Read the model definition and answer for the solid it produces. Units are mm, in the model's axes. Face numbers are marked on the shaded views. A direction names the side the tool comes from. Coordinates: 2 decimals unless noted, no trailing zeros. Order: outer loops, then holes, each group sorted by start corner. A loop starts at its lowest first (then second) coordinate and runs counter-clockwise, first axis right, second up. Notation, with made-up numbers: (52.5, -2.75) -> (105.5, -2.75) arc R18 cw to (105.5, 21.25) -> close; hole circle Ø6 at (-8.5, -17). An arc over 180 degrees is marked (long way). Answer as a JSON object with one key per item and string values. Group by question number.
1) Section D-D on y = 10.5 is taken. Determine the outline of the cut face in (x, z).
2) Consider L1, parallel to Z at x = 5, y = 23; L2, parallel to Y at x = 10.5, z = -26; L3, parallel to Y at x = -13, z = -24.5. Determine where each line is inside the solid, lowest interval first.
3) A tool of negligible diameter and unlimited length cuts with its end or side. For the marked faces 4 and 5, from which of +Z, -Z, +X, -X, +Y, -Y can it reach the whole face along a straight path? Write none if from no direction.
4) Determine the mould class of the marked faces 1, 2 and 3 for opening direction Z: released by +Z, released by -Z, zero draft, split by the parting line, or undercut.
5) Section C-C on z = 26 is taken. Determine the outline of the cut face in (x, y), and give its area (3 significant figures).
6) Section A-A on z = -10 is taken. Determine the outline of the cut face in (x, y).
7) Section B-B on x = -16.5 is taken. Determine the outline of the cut face in (y, z), and give its area (3 significant figures).
8) Given pin 1 (6 mm diameter, centred on y = 34.5, z = -14, fed in from -X); pin 2 (1.7 mm diameter, centred on y = 59, z = 9, fed in from -X); pin 3 (0.8 mm diameter, centred on y = 20, z = 29, fed in from -X), each flat-ended and moving along its own axis, determine where each tip first touches the part or whether it passes through.
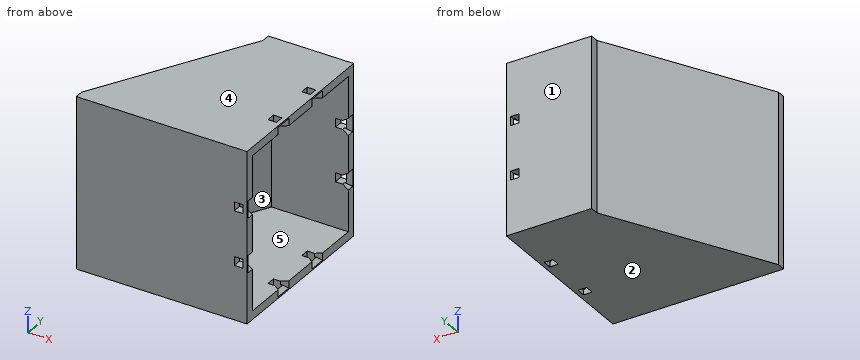
from build123d import *

# Parameters (mm, degrees)
SKETCH_1_W                    = 60
SKETCH_1_H                    = 60
EXTRUDE_1_DEPTH               = 3
SKETCH_2_W                    = 30
SKETCH_2_H                    = 60
EXTRUDE_2_DEPTH               = 3
EXTRUDE_3_DEPTH               = 3
EXTRUDE_4_DEPTH               = 3
SKETCH_8_W                    = 3
SKETCH_8_H                    = 3.1
CUT_EXTRUDE_2_DEPTH           = 91.000000167
SKETCH_9_W                    = 3
SKETCH_9_H                    = 3.1
CUT_EXTRUDE_3_DEPTH           = 74.484692447
SKETCH_7_W                    = 6
SKETCH_7_H                    = 5
CUT_EXTRUDE_1_DEPTH           = 2
CUT_EXTRUDE_1_DRAFT           = -36
SKETCH_7_W_2                  = 5
SKETCH_7_H_2                  = 6
CUT_EXTRUDE_1_PROFILE_2_DEPTH = 2
CUT_EXTRUDE_1_PROFILE_2_DRAFT = -36
CUT_EXTRUDE_1_PROFILE_3_DEPTH = 2
CUT_EXTRUDE_1_PROFILE_3_DRAFT = -36
CUT_EXTRUDE_1_PROFILE_4_DEPTH = 2
CUT_EXTRUDE_1_PROFILE_4_DRAFT = -36
CUT_EXTRUDE_1_PROFILE_5_DEPTH = 2
CUT_EXTRUDE_1_PROFILE_5_DRAFT = -36
CUT_EXTRUDE_1_PROFILE_6_DEPTH = 2
CUT_EXTRUDE_1_PROFILE_6_DRAFT = -36
CUT_EXTRUDE_1_PROFILE_7_DEPTH = 2
CUT_EXTRUDE_1_PROFILE_7_DRAFT = -36
CUT_EXTRUDE_1_PROFILE_8_DEPTH = 2
CUT_EXTRUDE_1_PROFILE_8_DRAFT = -36


with BuildPart() as part:
    # Sketch 1 → Extrude 1 (new body)
    with BuildSketch(Plane(origin=(0, 0, 0), x_dir=(1, 0, 0), z_dir=(0, 1, 0))):
        Rectangle(SKETCH_1_W, SKETCH_1_H)
    extrude(amount=EXTRUDE_1_DEPTH)



with BuildPart() as body_2:
    # Sketch 2 → Extrude 2 (new body)
    with BuildSketch(Plane(origin=(0, 57, 0), x_dir=(1, 0, 0), z_dir=(0, 1, 0))):
        with Locations((15, 0)):
            Rectangle(SKETCH_2_W, SKETCH_2_H)
    extrude(amount=EXTRUDE_2_DEPTH)


with BuildPart() as part_1:
    add(part.part)

    add(body_2.part)  # Loft 1 merges body 2
    # Sketch 3 → Loft 1 section 0
    with BuildSketch(Plane.XZ.offset(-57)):
        with BuildLine():
            Line((0, 30), (3, 30))
            Line((3, 30), (3, -30))
            Line((3, -30), (0, -30))
            Line((0, -30), (0, 30))
        make_face()
    # Sketch 4 → Loft 1 section 1
    with BuildSketch(Plane(origin=(0, 3, 0), x_dir=(1, 0, 0), z_dir=(0, 1, 0))):
        with BuildLine():
            Line((-30, 30), (-27, 30))
            Line((-27, 30), (-27, -30))
            Line((-27, -30), (-30, -30))
            Line((-30, -30), (-30, 30))
        make_face()
    loft()

    # Sketch 5 → Extrude 3 (add)
    with BuildSketch(Plane.XY.offset(30)):
        Polygon((30, 57), (3, 57), (-27, 3), (30, 3), align=None)
    extrude(amount=-EXTRUDE_3_DEPTH)

    # Sketch 6 → Extrude 4 (add)
    with BuildSketch(Plane(origin=(0, 0, -30), x_dir=(-1, 0, 0), z_dir=(0, 0, -1))):
        Polygon((-30, 57), (-3, 57), (27, 3), (-30, 3), align=None)
    extrude(amount=-EXTRUDE_4_DEPTH)

    # Sketch 8 → Cut-Extrude 2 (cut, through all)
    with BuildSketch(Plane(origin=(0, 0, -30), x_dir=(-1, 0, 0), z_dir=(0, 0, -1))):
        with Locations((-27, 39.5)):
            Rectangle(SKETCH_8_W, SKETCH_8_H)
        with Locations((-27, 20.5)):
            Rectangle(SKETCH_8_W, SKETCH_8_H)
    extrude(amount=-CUT_EXTRUDE_2_DEPTH, mode=Mode.SUBTRACT)

    # Sketch 9 → Cut-Extrude 3 (cut, through all)
    with BuildSketch(Plane(origin=(0, 60, 0), x_dir=(1, 0, 0), z_dir=(0, 1, 0))):
        with Locations((27, 9.5)):
            Rectangle(SKETCH_9_W, SKETCH_9_H)
        with Locations((27, -9.5)):
            Rectangle(SKETCH_9_W, SKETCH_9_H)
    extrude(amount=-CUT_EXTRUDE_3_DEPTH, mode=Mode.SUBTRACT)


with BuildPart() as cut_extrude_1_tool:
    # Sketch 7 → Cut-Extrude 1 (with draft: the straight prism first)
    with BuildSketch(Plane(origin=(30, 0, 0), x_dir=(0, 0, -1), z_dir=(1, 0, 0))):
        with Locations((9.5, 3)):
            Rectangle(SKETCH_7_W, SKETCH_7_H)
    extrude(amount=-CUT_EXTRUDE_1_DEPTH)
    # Cut-Extrude 1: the draft: its side faces are tilted about the plane it starts from
    cut_extrude_1_sides = [cut_extrude_1_tool.faces().sort_by_distance(p)[0] for p in [
        (29, 3, -6.5),
        (29, 0.5, -9.5),
        (29, 3, -12.5),
        (29, 5.5, -9.5),
    ]]
    draft(cut_extrude_1_sides, Plane(origin=(30, 0, 0), x_dir=(0, 0, -1), z_dir=(1, 0, 0)), CUT_EXTRUDE_1_DRAFT)


with BuildPart() as part_2:
    add(part_1.part)

    # Cut-Extrude 1: cut by cut_extrude_1_tool
    add(cut_extrude_1_tool.part, mode=Mode.SUBTRACT)


with BuildPart() as cut_extrude_1_profile_2_tool:
    # Sketch 7 → Cut-Extrude 1 profile 2 (with draft: the straight prism first)
    with BuildSketch(Plane(origin=(30, 0, 0), x_dir=(0, 0, -1), z_dir=(1, 0, 0))):
        with Locations((27, 39.5)):
            Rectangle(SKETCH_7_W_2, SKETCH_7_H_2)
    extrude(amount=-CUT_EXTRUDE_1_PROFILE_2_DEPTH)
    # Cut-Extrude 1 profile 2: the draft: its side faces are tilted about the plane it starts from
    cut_extrude_1_profile_2_sides = [cut_extrude_1_profile_2_tool.faces().sort_by_distance(p)[0] for p in [
        (29, 36.5, -27),
        (29, 39.5, -29.5),
        (29, 42.5, -27),
        (29, 39.5, -24.5),
    ]]
    draft(cut_extrude_1_profile_2_sides, Plane(origin=(30, 0, 0), x_dir=(0, 0, -1), z_dir=(1, 0, 0)), CUT_EXTRUDE_1_PROFILE_2_DRAFT)


with BuildPart() as part_3:
    add(part_2.part)

    # Cut-Extrude 1 profile 2: cut by cut_extrude_1_profile_2_tool
    add(cut_extrude_1_profile_2_tool.part, mode=Mode.SUBTRACT)


with BuildPart() as cut_extrude_1_profile_3_tool:
    # Sketch 7 → Cut-Extrude 1 profile 3 (with draft: the straight prism first)
    with BuildSketch(Plane(origin=(30, 0, 0), x_dir=(0, 0, -1), z_dir=(1, 0, 0))):
        with Locations((27, 20.5)):
            Rectangle(SKETCH_7_W_2, SKETCH_7_H_2)
    extrude(amount=-CUT_EXTRUDE_1_PROFILE_3_DEPTH)
    # Cut-Extrude 1 profile 3: the draft: its side faces are tilted about the plane it starts from
    cut_extrude_1_profile_3_sides = [cut_extrude_1_profile_3_tool.faces().sort_by_distance(p)[0] for p in [
        (29, 23.5, -27),
        (29, 20.5, -24.5),
        (29, 17.5, -27),
        (29, 20.5, -29.5),
    ]]
    draft(cut_extrude_1_profile_3_sides, Plane(origin=(30, 0, 0), x_dir=(0, 0, -1), z_dir=(1, 0, 0)), CUT_EXTRUDE_1_PROFILE_3_DRAFT)


with BuildPart() as part_4:
    add(part_3.part)

    # Cut-Extrude 1 profile 3: cut by cut_extrude_1_profile_3_tool
    add(cut_extrude_1_profile_3_tool.part, mode=Mode.SUBTRACT)


with BuildPart() as cut_extrude_1_profile_4_tool:
    # Sketch 7 → Cut-Extrude 1 profile 4 (with draft: the straight prism first)
    with BuildSketch(Plane(origin=(30, 0, 0), x_dir=(0, 0, -1), z_dir=(1, 0, 0))):
        with Locations((-9.5, 3)):
            Rectangle(SKETCH_7_W, SKETCH_7_H)
    extrude(amount=-CUT_EXTRUDE_1_PROFILE_4_DEPTH)
    # Cut-Extrude 1 profile 4: the draft: its side faces are tilted about the plane it starts from
    cut_extrude_1_profile_4_sides = [cut_extrude_1_profile_4_tool.faces().sort_by_distance(p)[0] for p in [
        (29, 3, 6.5),
        (29, 5.5, 9.5),
        (29, 3, 12.5),
        (29, 0.5, 9.5),
    ]]
    draft(cut_extrude_1_profile_4_sides, Plane(origin=(30, 0, 0), x_dir=(0, 0, -1), z_dir=(1, 0, 0)), CUT_EXTRUDE_1_PROFILE_4_DRAFT)


with BuildPart() as part_5:
    add(part_4.part)

    # Cut-Extrude 1 profile 4: cut by cut_extrude_1_profile_4_tool
    add(cut_extrude_1_profile_4_tool.part, mode=Mode.SUBTRACT)


with BuildPart() as cut_extrude_1_profile_5_tool:
    # Sketch 7 → Cut-Extrude 1 profile 5 (with draft: the straight prism first)
    with BuildSketch(Plane(origin=(30, 0, 0), x_dir=(0, 0, -1), z_dir=(1, 0, 0))):
        with Locations((-27, 20.5)):
            Rectangle(SKETCH_7_W_2, SKETCH_7_H_2)
    extrude(amount=-CUT_EXTRUDE_1_PROFILE_5_DEPTH)
    # Cut-Extrude 1 profile 5: the draft: its side faces are tilted about the plane it starts from
    cut_extrude_1_profile_5_sides = [cut_extrude_1_profile_5_tool.faces().sort_by_distance(p)[0] for p in [
        (29, 23.5, 27),
        (29, 20.5, 29.5),
        (29, 17.5, 27),
        (29, 20.5, 24.5),
    ]]
    draft(cut_extrude_1_profile_5_sides, Plane(origin=(30, 0, 0), x_dir=(0, 0, -1), z_dir=(1, 0, 0)), CUT_EXTRUDE_1_PROFILE_5_DRAFT)


with BuildPart() as part_6:
    add(part_5.part)

    # Cut-Extrude 1 profile 5: cut by cut_extrude_1_profile_5_tool
    add(cut_extrude_1_profile_5_tool.part, mode=Mode.SUBTRACT)


with BuildPart() as cut_extrude_1_profile_6_tool:
    # Sketch 7 → Cut-Extrude 1 profile 6 (with draft: the straight prism first)
    with BuildSketch(Plane(origin=(30, 0, 0), x_dir=(0, 0, -1), z_dir=(1, 0, 0))):
        with Locations((-27, 39.5)):
            Rectangle(SKETCH_7_W_2, SKETCH_7_H_2)
    extrude(amount=-CUT_EXTRUDE_1_PROFILE_6_DEPTH)
    # Cut-Extrude 1 profile 6: the draft: its side faces are tilted about the plane it starts from
    cut_extrude_1_profile_6_sides = [cut_extrude_1_profile_6_tool.faces().sort_by_distance(p)[0] for p in [
        (29, 36.5, 27),
        (29, 39.5, 24.5),
        (29, 42.5, 27),
        (29, 39.5, 29.5),
    ]]
    draft(cut_extrude_1_profile_6_sides, Plane(origin=(30, 0, 0), x_dir=(0, 0, -1), z_dir=(1, 0, 0)), CUT_EXTRUDE_1_PROFILE_6_DRAFT)


with BuildPart() as part_7:
    add(part_6.part)

    # Cut-Extrude 1 profile 6: cut by cut_extrude_1_profile_6_tool
    add(cut_extrude_1_profile_6_tool.part, mode=Mode.SUBTRACT)


with BuildPart() as cut_extrude_1_profile_7_tool:
    # Sketch 7 → Cut-Extrude 1 profile 7 (with draft: the straight prism first)
    with BuildSketch(Plane(origin=(30, 0, 0), x_dir=(0, 0, -1), z_dir=(1, 0, 0))):
        with Locations((-9.5, 57)):
            Rectangle(SKETCH_7_W, SKETCH_7_H)
    extrude(amount=-CUT_EXTRUDE_1_PROFILE_7_DEPTH)
    # Cut-Extrude 1 profile 7: the draft: its side faces are tilted about the plane it starts from
    cut_extrude_1_profile_7_sides = [cut_extrude_1_profile_7_tool.faces().sort_by_distance(p)[0] for p in [
        (29, 57, 6.5),
        (29, 59.5, 9.5),
        (29, 57, 12.5),
        (29, 54.5, 9.5),
    ]]
    draft(cut_extrude_1_profile_7_sides, Plane(origin=(30, 0, 0), x_dir=(0, 0, -1), z_dir=(1, 0, 0)), CUT_EXTRUDE_1_PROFILE_7_DRAFT)


with BuildPart() as part_8:
    add(part_7.part)

    # Cut-Extrude 1 profile 7: cut by cut_extrude_1_profile_7_tool
    add(cut_extrude_1_profile_7_tool.part, mode=Mode.SUBTRACT)


with BuildPart() as cut_extrude_1_profile_8_tool:
    # Sketch 7 → Cut-Extrude 1 profile 8 (with draft: the straight prism first)
    with BuildSketch(Plane(origin=(30, 0, 0), x_dir=(0, 0, -1), z_dir=(1, 0, 0))):
        with Locations((9.5, 57)):
            Rectangle(SKETCH_7_W, SKETCH_7_H)
    extrude(amount=-CUT_EXTRUDE_1_PROFILE_8_DEPTH)
    # Cut-Extrude 1 profile 8: the draft: its side faces are tilted about the plane it starts from
    cut_extrude_1_profile_8_sides = [cut_extrude_1_profile_8_tool.faces().sort_by_distance(p)[0] for p in [
        (29, 57, -6.5),
        (29, 54.5, -9.5),
        (29, 57, -12.5),
        (29, 59.5, -9.5),
    ]]
    draft(cut_extrude_1_profile_8_sides, Plane(origin=(30, 0, 0), x_dir=(0, 0, -1), z_dir=(1, 0, 0)), CUT_EXTRUDE_1_PROFILE_8_DRAFT)


with BuildPart() as part_9:
    add(part_8.part)

    # Cut-Extrude 1 profile 8: cut by cut_extrude_1_profile_8_tool
    add(cut_extrude_1_profile_8_tool.part, mode=Mode.SUBTRACT)


solid = part_9.part
Worked answers:
{
 "1": {"outline": "(-25.83, -30) -> (30, -30) -> (30, -27) -> (-22.83, -27) -> (-22.83, 27) -> (30, 27) -> (30, 30) -> (-25.83, 30) -> close"},
 "2": {"L1": "z = -30 to -27, 27 to 30", "L2": "y = 0 to 3, 57 to 60", "L3": "y = 0 to 3, 28.2 to 33.6"},
 "3": {"face 4": "+Z, +X, -X, +Y, -Y", "face 5": "+X"},
 "4": {"face 1": "zero draft", "face 2": "released by -Z", "face 3": "undercut"},
 "5": {"outline": "(-30, 0) -> (30, 0) -> (30, 3) -> (-27, 3) -> (3, 57) -> (30, 57) -> (30, 60) -> (0, 60) -> (0, 57) -> (-30, 3) -> close", "area": "432 mm²"},
 "6": {"outline": "(-30, 0) -> (25.5, 0) -> (25.5, 3) -> (-27, 3) -> (3, 57) -> (25.5, 57) -> (25.5, 60) -> (0, 60) -> (0, 57) -> (-30, 3) -> close; (28.5, 0) -> (30, 0) -> (30, 0.5) -> (28.5, 1.59) -> close; (28.5, 58.41) -> (30, 59.5) -> (30, 60) -> (28.5, 60) -> close"},
 "7": {"outline": "(0, -30) -> (27.3, -30) -> (27.3, 30) -> (0, 30) -> close; hole (3, -27) -> (21.9, -27) -> (21.9, 27) -> (3, 27) -> close", "area": "617 mm²"},
 "8": {"pin 1": "stops at x = -14.17", "pin 2": "stops at x = 0", "pin 3": "stops at x = -20.78"}
}
